The model under review builds one solid part; all positions refer to its coordinate system, in mm. A direction names the side the tool comes from. Coordinates: 2 decimals unless noted, no trailing zeros. Loops run counter-clockwise (first coordinate to the right, second up) from the corner with the lowest first, then second, coordinate; pieces in that order, holes last. Notation, with made-up numbers: M 12,34 L 49,34 A20 cw 49,42 Z; hole C 73,19.25 d8. An arc over 180 degrees is marked long. Use one line per item in the form item = value.
```python
from build123d import *

# Parameters (mm, degrees)
SKETCH_1_W           = 27
SKETCH_1_H           = 10.8
EXTRUDE_1_DEPTH      = 12
SKETCH_2_W           = 3.9
SKETCH_2_H           = 3.9
CUT_EXTRUDE_2_DEPTH  = 10.5
FILLET_3_R           = 1.5
FILLET_4_R           = 1.5
SKETCH_3_R           = 1.1
CUT_EXTRUDE_3_DEPTH  = 2.1
SKETCH_4_W           = 27
SKETCH_4_H           = 10.8
SKETCH_4_W_2         = 19.2
SKETCH_4_H_2         = 8
CUT_EXTRUDE_4_DEPTH  = 4
SKETCH_5_W           = 9
SKETCH_5_H           = 3
EXTRUDE_2_DEPTH      = 2.108
EXTRUDE_2_DEPTH_BACK = 3


with BuildPart() as part:
    # 스케치1 → 보스-돌출1 (new body)
    with BuildSketch(Plane.XY):
        with Locations((-12.645283423, 9.45123242)):
            Rectangle(SKETCH_1_W, SKETCH_1_H)
    extrude(amount=EXTRUDE_1_DEPTH)

    # 스케치2 → 컷-돌출2 (cut)
    with BuildSketch(Plane.XY.offset(12)):
        with Locations((-24.195283423, 12.90123242)):
            Rectangle(SKETCH_2_W, SKETCH_2_H)
        with Locations((-1.095283423, 6.00123242)):
            Rectangle(SKETCH_2_W, SKETCH_2_H)
    extrude(amount=-CUT_EXTRUDE_2_DEPTH, mode=Mode.SUBTRACT)

    # 필렛3
    fillet_3_edges = [part.edges().sort_by_distance(p)[0] for p in [
        (-22.245283423, 10.95123242, 6.75),
    ]]
    fillet(fillet_3_edges, radius=FILLET_3_R)

    # 필렛4
    fillet_4_edges = [part.edges().sort_by_distance(p)[0] for p in [
        (-3.045283423, 7.95123242, 6.75),
    ]]
    fillet(fillet_4_edges, radius=FILLET_4_R)

    # 스케치3 → 컷-돌출3 (cut)
    with BuildSketch(Plane.XY.offset(1.5)):
        with Locations((-24.345283423, 12.75123242)):
            Circle(SKETCH_3_R)
        with Locations((-0.945283423, 6.15123242)):
            Circle(SKETCH_3_R)
    extrude(amount=-CUT_EXTRUDE_3_DEPTH, mode=Mode.SUBTRACT)

    # 스케치4 → 컷-돌출4 (cut)
    with BuildSketch(Plane.XY.offset(12)):
        with Locations((-12.645283423, 9.45123242)):
            Rectangle(SKETCH_4_W, SKETCH_4_H)
        with Locations((-12.645283423, 9.45123242)):
            Rectangle(SKETCH_4_W_2, SKETCH_4_H_2, mode=Mode.SUBTRACT)
    extrude(amount=-CUT_EXTRUDE_4_DEPTH, mode=Mode.SUBTRACT)

    # 스케치5 → 보스-돌출2 (add, two sides)
    with BuildSketch(Plane(origin=(0, 0, 0), x_dir=(-1, 0, 0), z_dir=(0, 0, -1))) as extrude_2_sk:
        with Locations((4.495283423, 15.75123242)):
            Rectangle(SKETCH_5_W, SKETCH_5_H)
    extrude(amount=EXTRUDE_2_DEPTH)
    extrude(extrude_2_sk.sketch, amount=-EXTRUDE_2_DEPTH_BACK)


solid = part.part
```
1. Add section D-D (z = 4.75). State the section outline as (x, y) points.
Response values:
outline = M -26.15,4.05 L -3.05,4.05 L -3.05,6.45 A1.5 cw -1.55,7.95 L 0.85,7.95 L 0.85,14.85 L -22.25,14.85 L -22.25,12.45 A1.5 cw -23.75,10.95 L -26.15,10.95 Z
2. Add section A-A (x = -20.75). State the section outline as (y, z) points.
Response values:
outline = M 4.05,0 L 14.85,0 L 14.85,8 L 13.45,8 L 13.45,12 L 5.45,12 L 5.45,8 L 4.05,8 Z
3. Add section B-B (y = 9). State the section outline as (x, z) points, then the cut area to 3 significant figures.
Response values:
outline = M -26.15,0 L 0.85,0 L 0.85,8 L -3.05,8 L -3.05,12 L -22.25,12 L -22.25,8 L -26.15,8 Z
area = 293 mm^2
4. Wall thickness on line 1 along Y through (x, z) = (-17.25, 9.5); line 2 along Z through (x, y) = (-3, 13); line 3 along Z through (x, y) = (-7.25, 16.5): over which ranges is each line inside the solid? List them lowest first. Write a range as from..to.
Response values:
line_1 = 5.45..13.45
line_2 = 0..8
line_3 = -2.11..3
5. Machinability: for faces 1 (the face through (-25, 10.951, 5)), 2 (the face through (-13, 13.451, 10)), 3 (the face through (-13, 5.451, 10)), 4 (the face through (-13, 10, 12)), 5 (the face through (0, 7.951, 5)), which of the approach directions +Z, -Z, +X, -X, +Y, -Y give a long, thin tool a straight path to every point of the face, cutting with its end or side? Answer none if there is none.
Response values:
face_1 = +Z, -X, +Y
face_2 = +Z, +X, -X, +Y
face_3 = +Z, +X, -X, -Y
face_4 = +Z, +X, -X, +Y, -Y
face_5 = +Z, +X, -Y
6. Insertion check: P1, Ø1.5, axis at x = -6, z = 9.5, coming from the +Y side; P2, Ø3.5, axis at x = -24.35, y = 12.75, coming from the +Z side; P3, Ø1.2, axis at x = -2.5, y = 15.5, coming from the +Z side. Each pin has a flat end and moves straight along its axis. Give the tip position at first contact, or say it passes through.
Response values:
P1 = 13.45
P2 = 1.5
P3 = 3
7. Add section C-C (y = 12). State the section outline as (x, z) points.
Response values:
outline = M -26.15,0 L -25.15,0 L -25.15,1.5 L -26.15,1.5 Z; M -23.54,0 L 0.85,0 L 0.85,8 L -3.05,8 L -3.05,12 L -22.25,12 L -22.25,8 L -22.31,8 L -22.31,1.5 L -23.54,1.5 Z
8. The part is to be moulded in two halves that separate along X. For faces 6 (the face through (-26.145, 8, 4)), 7 (the face through (-23.838, 11.775, 0.76)), 8 (the face through (-4, 14.251, -1)), 9 (the face through (-2.62, 7.5, 4.7)), say which applies: pulls with the +X half, pulls with the -X half, needs draft (parallel to the pull), parting line crosses it, or undercut.
Response values:
face_6 = pulls with the -X half
face_7 = undercut
face_8 = needs draft
face_9 = pulls with the +X half
